Autodesk Fusion 360 part; units mm, degrees
sketch "スケッチ1" plane through (0, 0, 0) normal (0, 0, 1) x (1, 0, 0)
  circle A0 centre (0, 0) radius 2.45
  circle A1 centre (0, 0) radius 3.5
  line L0 (-3.5, 0) -> (3.5, 0) construction
  line L1 (0, 3.5) -> (0, -3.5) construction
  line L2 (-0.35, 2.4249) -> (0, 2.25)
  line L3 (0.35, 2.4249) -> (0, 2.25)
  line L4 (-0.35, 2.4249) -> (0.35, 2.4249) construction
  line L5 (0, 2.45) -> (0, 2.25) construction
  circle A2 centre (0, 0) radius 1.25
  line L6 (0, 3.5) -> (0, 16) construction
  line L7 (-2.75, 2.1651) -> (2.75, 2.1651) construction
  circle A3 centre (0, 14.1) radius 1.9
  line L8 (-1.9, 14.1) -> (1.9, 14.1) construction
  line L9 (-1.9, 14.1) -> (-2.75, 2.1651)
  line L10 (1.9, 14.1) -> (2.75, 2.1651)
  circle A4 centre (0, 14.8) radius 0.45
  circle A5 centre (0, 12.7) radius 0.45
  circle A6 centre (0, 10.6) radius 0.45
  circle A7 centre (0, 8.5) radius 0.45
  circle A8 centre (0, 6.4) radius 0.45
  circle A9 centre (0, 4.3) radius 0.45
  circle A10 centre (0, 0) radius 2.35
  dimension "d1" = 4.9
  dimension "d2" = 7
  dimension "d3" = 0.2
  dimension "d4" = 0.7
  dimension "d5" = 2.5
  dimension "d7" = 3.8
  dimension "d8" = 19.5
  dimension "d9" = 5.5
  dimension "d10" = 0.9
  dimension "d12" = 2.1
  dimension "d13" = 2.1
  dimension "d14" = 2.1
  dimension "d15" = 2.1
  dimension "d16" = 2.1
  dimension "d18" = 4.7
  dimension "d21" = 1.2
extrude "押し出し1" add sketch "スケッチ1" along normal blind 1 contours A0 L2 L3 A10 | A0 L2 L3 A10 | A1 | A1 A3 L9 L10 | A3
extrude "押し出し2" add sketch "スケッチ1" along normal blind 1.5 contours A1 A3 L9 L10 | A3
extrude "押し出し3" add sketch "スケッチ1" along normal blind 0.8 from surface at 1 contours A0 L2 L3 A10 | A0 L2 L3 A10 | L2 L3 A10 | L2 L3 A10 | A1
extrude "押し出し4" add sketch "スケッチ1" along normal blind 2 from surface at 1.8 contours A1
extrude "押し出し5" add sketch "スケッチ1" along normal blind 2 from surface at 1.8 contours A0 L2 L3 A10 | L2 L3 A10 picked at (-0.3559, 2.3522) picked at (0, 2.3161)
pattern_circular "C パターン1" count 22 over 360 about axis through (0, 0, 1.75) along (0, 0, 1) of "押し出し5"
Geometry: final body of the model. Coordinates: model frame, mm. A direction names the side the tool comes from. Round coordinates to 2 decimals unless told otherwise and drop trailing zeros. Write each loop counter-clockwise with the first axis right and the second up, starting at its lowest first coordinate (ties: lowest second). Pieces come first, ordered by that corner, then holes.
Item 1: Set-up query: faces 5 (the face through (0, 16, 1)), 6 (the face through (3.163, -1.499, 1.873)), 7 (the face through (1, -1, 1)). Return all of +Z, -Z, +X, -X, +Y, -Y with unobstructed straight access to the full face (end or side cutting, diameter ignored); none if empty.
Item 2: Section query B-B (z = 0.55). Return loops of the section in (x, y).
Item 3: Section query D-D (y = 11.5). Return loops of the section in (x, z).
Item 4: Section query A-A (y = 6.4). Return loops of the section in (x, z), plus the area to 3 significant figures.
Item 5: Material intervals for L1, parallel to Y at x = 0, z = 1.6; L2, parallel to Z at x = 1, y = 3.75; L3, parallel to X at y = 8.75, z = 1, sorted ascending.
Item 6: Section query C-C (y = 4.3). Return loops of the section in (x, z).
Item 7: Mould query, pull axis X, two halves, no side actions, for faces 1 (the face through (-2.32, 8.22, 0.74)), 2 (the face through (-0.1, 6.84, 0.74)), 3 (the face through (1, 6, 0)), 4 (the face through (2.32, 8.22, 0.74)). Classes: +X half, -X half, draft (parallel to the pull), parting line (faces both ways), or undercut.
Item 8: Pin query (flat end, axial travel): P1, Ø4, axis at x = -1.5, y = 0, coming from the -Z side; P2, Ø1, axis at y = 3, z = 1.5, coming from the -X side; P3, Ø1.5, axis at x = 0, y = 0, coming from the +Z side. Return the tip coordinate at first contact, or that it passes through.
Completed:
1. face 5: +Z, -Z, +Y
1. face 6: +Z
1. face 7: -Z
2. outline: (-2.75, 2.17) arc R3.5 ccw (long way) to (2.75, 2.17) - (1.9, 14.1) arc R1.9 ccw to (-1.9, 14.1) - close; hole circle Ø4.7 at (0, 0); hole circle Ø0.9 at (0, 4.3); hole circle Ø0.9 at (0, 6.4); hole circle Ø0.9 at (0, 8.5); hole circle Ø0.9 at (0, 10.6); hole circle Ø0.9 at (0, 12.7); hole circle Ø0.9 at (0, 14.8)
3. outline: (-2.09, 0) - (2.09, 0) - (2.09, 1.5) - (-2.09, 1.5) - close
4. outline: (-2.45, 0) - (-0.45, 0) - (-0.45, 1.5) - (-2.45, 1.5) - close; (0.45, 0) - (2.45, 0) - (2.45, 1.5) - (0.45, 1.5) - close
4. area: 6.00 mm2
5. L1: y = -3.5 to -1.25, 1.25 to 3.5
5. L2: z = 0 to 1.5
5. L3: x = -2.28 to -0.37, 0.37 to 2.28
6. outline: (-2.6, 0) - (-0.45, 0) - (-0.45, 1.5) - (-2.6, 1.5) - close; (0.45, 0) - (2.6, 0) - (2.6, 1.5) - (0.45, 1.5) - close
7. face 1: -X half
7. face 2: undercut
7. face 3: draft
7. face 4: +X half
8. P1: stops at z = 0
8. P2: stops at x = -2.73
8. P3: passes through
